The model under review builds one solid part; all positions refer to its coordinate system, in mm. Round coordinates to 2 decimals unless told otherwise and drop trailing zeros. Order: outer loops, then holes, each group sorted by start corner. A loop starts at its lowest first (then second) coordinate and runs counter-clockwise, first axis right, second up. Notation, with made-up numbers: (26, 51) -> (59, 51) arc R17 ccw to (59, 60) -> close; hole circle Ø1 at (-39.75, 82.5). An arc over 180 degrees is marked (long way). Use a Markdown table: item, result. Add a question column.
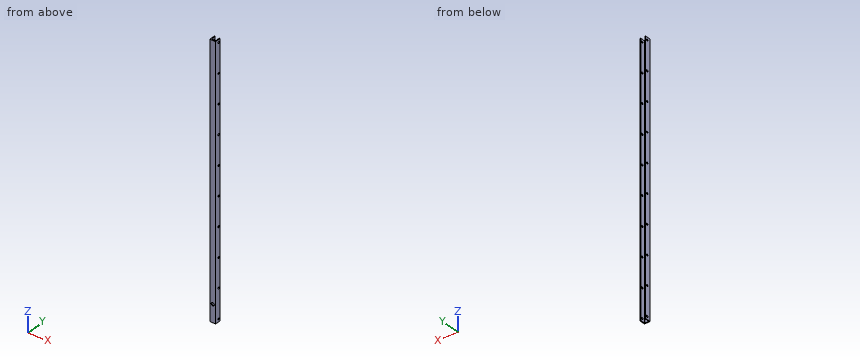
```python
from build123d import *

# Parameters (mm, degrees)
BOSS_EXTRUDE1_DEPTH = 460
FILLET1_R           = 0.5
FILLET2_R           = 0.1
SKETCH2_R           = 1.6
CUT_EXTRUDE1_DEPTH  = 461.21733996
SKETCH4_R           = 2.7
CUT_EXTRUDE2_DEPTH  = 461.135849505


with BuildPart() as part:
    # Sketch1 → Boss-Extrude1 (new body)
    with BuildSketch(Plane.XY):
        Polygon((-5, 0), (5, 0), (5, 10), (3.5, 10), (3.5, 1.5), (-3.5, 1.5), (-3.5, 10), (-5, 10), align=None)
    extrude(amount=BOSS_EXTRUDE1_DEPTH)

    # Fillet1
    fillet1_edges = [part.edges().sort_by_distance(p)[0] for p in [
        (-3.5, 1.5, 230),
        (3.5, 1.5, 230),
    ]]
    fillet(fillet1_edges, radius=FILLET1_R)

    # Fillet2
    fillet2_edges = [part.edges().sort_by_distance(p)[0] for p in [
        (5, 0, 230),
        (-5, 0, 230),
        (-5, 10, 230),
        (-3.5, 10, 230),
        (3.5, 10, 230),
        (5, 10, 230),
    ]]
    fillet(fillet2_edges, radius=FILLET2_R)

    # Sketch2 → Cut-Extrude1 (cut, through all)
    with BuildSketch(Plane.ZY.offset(5)):
        with Locations((5, 6.7)):
            Circle(SKETCH2_R)
        with Locations((55, 6.7)):
            Circle(SKETCH2_R)
        with Locations((105, 6.7)):
            Circle(SKETCH2_R)
        with Locations((155, 6.7)):
            Circle(SKETCH2_R)
        with Locations((205, 6.7)):
            Circle(SKETCH2_R)
        with Locations((255, 6.7)):
            Circle(SKETCH2_R)
        with Locations((305, 6.7)):
            Circle(SKETCH2_R)
        with Locations((355, 6.7)):
            Circle(SKETCH2_R)
        with Locations((405, 6.7)):
            Circle(SKETCH2_R)
        with Locations((455, 6.7)):
            Circle(SKETCH2_R)
        with Locations((505, 6.7)):
            Circle(SKETCH2_R)
    extrude(amount=-CUT_EXTRUDE1_DEPTH, mode=Mode.SUBTRACT)

    # Sketch4 → Cut-Extrude2 (cut, through all)
    with BuildSketch(Plane.XZ):
        with Locations(Location((0, 30, 0), (0, 0, 270))):
            Circle(SKETCH4_R)
    extrude(amount=-CUT_EXTRUDE2_DEPTH, mode=Mode.SUBTRACT)


solid = part.part
```
Q1. Add section A-A (x = 0). Write out the cut boundary in (y, z), then the cut area to 3 significant figures.
Q2. Insertion check: pin 1 (1.8 mm diameter, centred on x = 0, z = 185.5, fed in from +Y). The pin has a flat end and moves straight along its axis. Give the tip position at first contact, or say it passes through.
Q3. Wall thickness on line 1 (Y direction, x = -4.5, z = 355); line 2 (X direction, y = 5, z = 404); line 3 (Y direction, x = 3, z = 248.5): over which ranges is each line inside the solid? List them lowest first. Write a range as [from, to].
Q4. Add section B-B (y = 3.5). Write out the cut boundary in (x, z), then the cut area to 3 significant figures.
Q5. Add section C-C (z = 72.5). Write out the cut boundary in (x, y), then the cut area to 3 significant figures.
Report:
| question | item | result |
|---|---|---|
| 1 | outline | (0, 0) -> (1.5, 0) -> (1.5, 27.3) -> (0, 27.3) -> close; (0, 32.7) -> (1.5, 32.7) -> (1.5, 460) -> (0, 460) -> close |
| 1 | area | 682 mm² |
| 2 | pin 1 | stops at y = 1.5 |
| 3 | line 1 | y = [0, 5.1], [8.3, 10] |
| 3 | line 2 | x = [-5, -3.5], [3.5, 5] |
| 3 | line 3 | y = [0, 1.5] |
| 4 | outline | (-5, 0) -> (-3.5, 0) -> (-3.5, 460) -> (-5, 460) -> close; (3.5, 0) -> (5, 0) -> (5, 460) -> (3.5, 460) -> close |
| 4 | area | 1,380 mm² |
| 5 | outline | (-5, 0.1) arc R0.1 ccw to (-4.9, 0) -> (4.9, 0) arc R0.1 ccw to (5, 0.1) -> (5, 9.9) arc R0.1 ccw to (4.9, 10) -> (3.6, 10) arc R0.1 ccw to (3.5, 9.9) -> (3.5, 2) arc R0.5 cw to (3, 1.5) -> (-3, 1.5) arc R0.5 cw to (-3.5, 2) -> (-3.5, 9.9) arc R0.1 ccw to (-3.6, 10) -> (-4.9, 10) arc R0.1 ccw to (-5, 9.9) -> close |
| 5 | area | 40.6 mm² |
